Geometry check sheet. Reference: the model listing, model coordinates, mm. A direction names the side the tool comes from. Round coordinates to 2 decimals unless told otherwise and drop trailing zeros. Loops run counter-clockwise (first coordinate to the right, second up) from the corner with the lowest first, then second, coordinate; pieces in that order, holes last. Notation, with made-up numbers: (12.5, 49) - (27.5, 49) arc R21 ccw to (27.5, 79) - close; hole circle Ø9 at (76, -33.75). An arc over 180 degrees is marked (long way). Answer as CSV lines item,"result". Start each with the question number.
1) Cross-section at C-C on z = -7.1. Record the boundary of the cut face in (x, y) (3 decimals).
2) Cross-section at D-D on y = 5.5. Record the boundary of the cut face in (x, z), and give its area (3 significant figures).
3) Depth check by flat-ended pin: P1, Ø8, axis at y = 11.5, z = -7, coming from the -X side; P2, Ø3, axis at x = -1.5, z = 10.5, coming from the +Y side; P3, Ø1, axis at y = 3, z = -3.5, coming from the +X side; P4, Ø0.6, axis at x = -2, y = 3, coming from the -Z side. Enter the tip coordinate at first touch or a pass-through.
4) Draft check along Z on faces 4 (the cylindrical face through (-14.63, 1.01, 3.44)), 5 (the cylindrical face through (-13.887, 0.986, 10.648)), 6 (the flat face through (-4, 4, -4)). Enter one of: released by +Z, released by -Z, zero draft, split by the parting line, or undercut.
5) Cross-section at A-A on y = 3. Record the boundary of the cut face in (x, z), and give its area (3 significant figures).
6) Thickness scan on line 1 along Z through (x, y) = (-2, 2.1); line 2 along Z through (x, y) = (-13.5, 1.25); line 3 along X through (y, z) = (1.35, -4.1). Record the ranges inside material, lowest first.
7) Cross-section at B-B on y = 9. Record the boundary of the cut face in (x, z).
8) Access from +Z, -Z, +X, -X, +Y, -Y to the whole of each face (thin tool, end or side, straight path). Record for faces 1 (the cylindrical face through (-1, 3, -0.7)), 2 (the cylindrical face through (4.5, 9, 1.1)), 3 (the cylindrical face through (14.049, 1.014, 8.166)).
from build123d import *

# Parameters (mm, degrees)
SKETCH1_R                                       = 17.5
BOSS_EXTRUDE1_DEPTH                             = 2
CUT_EXTRUDE1_DEPTH                              = 3
CIRPATTERN1_COUNT                               = 6
SKETCH3_W                                       = 13.5
SKETCH3_H                                       = 16.4
BOSS_EXTRUDE2_DEPTH                             = 17.5
SKETCH4_W                                       = 13.5
SKETCH4_H                                       = 8.2
CUT_EXTRUDE2_DEPTH                              = 11.5
CUT_EXTRUDE3_DEPTH                              = 26.7
CUT_EXTRUDE4_DEPTH                              = 8.2
F_1_5MM_DOWEL_HOLE1_D                           = 1.5
F_1_5MM_DOWEL_HOLE1_DEPTH                       = 5
F_1_5MM_DOWEL_HOLE1_TIP                         = 0.450645464
F_1_5MM_DOWEL_HOLE2_D                           = 1.5
F_1_5MM_DOWEL_HOLE2_DEPTH                       = 3
F_1_5MM_DOWEL_HOLE2_TIP                         = 0.450645464
F_1_5MM_DOWEL_HOLE4_D                           = 1.5
F_1_5MM_DOWEL_HOLE4_DEPTH                       = 5
F_1_5MM_DOWEL_HOLE4_TIP                         = 0.450645464
F_1_5MM_DOWEL_HOLE3_D                           = 1.5
F_1_5MM_DOWEL_HOLE3_DEPTH                       = 5
F_1_5MM_DOWEL_HOLE3_TIP                         = 0.450645464
SKETCH16_R                                      = 1
CUT_EXTRUDE7_DEPTH                              = 14.5
CSK_FOR_M2_FLAT_HEAD_MACHINE_SCREW2_D           = 2.4
CSK_FOR_M2_FLAT_HEAD_MACHINE_SCREW2_CSINK_D     = 4.4
CSK_FOR_M2_FLAT_HEAD_MACHINE_SCREW2_CSINK_ANGLE = 90
CUT_EXTRUDE6_DEPTH                              = 11.5


with BuildPart() as part:
    # Sketch1 → Boss-Extrude1 (new body)
    with BuildSketch(Plane(origin=(0, 0, 0), x_dir=(1, 0, 0), z_dir=(0, 1, 0))):
        Circle(SKETCH1_R)
    extrude(amount=BOSS_EXTRUDE1_DEPTH)

    # Sketch2 → Cut-Extrude1 (cut, through all)
    with BuildSketch(Plane(origin=(0, 2, 0), x_dir=(1, 0, 0), z_dir=(0, 1, 0))):
        with BuildLine():
            ThreePointArc((3.378564976, 15.894898512), (0, 16.25), (-3.378564976, 15.894898512))
            ThreePointArc((-3.378564976, 15.894898512), (-4.341359863, 14.412324397), (-2.858785749, 13.44952951))
            ThreePointArc((-2.858785749, 13.44952951), (0, 13.75), (2.858785749, 13.44952951))
            ThreePointArc((2.858785749, 13.44952951), (4.341359863, 14.412324397), (3.378564976, 15.894898512))
        make_face()
    cut_extrude1 = extrude(amount=-CUT_EXTRUDE1_DEPTH, mode=Mode.SUBTRACT)

    # CirPattern1: Cut-Extrude1 ×6 about axis
    cirpattern1_axis = Axis((0, 0, 0), (0, 1, 0))
    for i in range(1, CIRPATTERN1_COUNT):
        add(cut_extrude1.rotate(cirpattern1_axis, i * 360 / CIRPATTERN1_COUNT), mode=Mode.SUBTRACT)

    # Sketch3 → Boss-Extrude2 (add)
    with BuildSketch(Plane(origin=(0, 2, 0), x_dir=(1, 0, 0), z_dir=(0, 1, 0))):
        Rectangle(SKETCH3_W, SKETCH3_H)
    extrude(amount=BOSS_EXTRUDE2_DEPTH)

    # Sketch4 → Cut-Extrude2 (cut)
    with BuildSketch(Plane(origin=(0, 19.5, 0), x_dir=(1, 0, 0), z_dir=(0, 1, 0))):
        with Locations((0, 4.1)):
            Rectangle(SKETCH4_W, SKETCH4_H)
    extrude(amount=-CUT_EXTRUDE2_DEPTH, mode=Mode.SUBTRACT)

    # Sketch5 → Cut-Extrude3 (cut, through all)
    with BuildSketch(Plane.XY.offset(8.2)):
        Polygon((-6.75, 19.5), (-6.75, 13.5), (0, 13.5), (0, 10.5), (6.75, 10.5), (6.75, 19.5), align=None)
    extrude(amount=-CUT_EXTRUDE3_DEPTH, mode=Mode.SUBTRACT)

    # Sketch6 → Cut-Extrude4 (cut)
    with BuildSketch(Plane(origin=(0, 0, -8.2), x_dir=(-1, 0, 0), z_dir=(0, 0, -1))):
        Polygon((6.75, 8), (6.75, 4), (0, 4), (0, 2), (-6.75, 2), (-6.75, 8), align=None)
    extrude(amount=-CUT_EXTRUDE4_DEPTH, mode=Mode.SUBTRACT)

    # Ø1.5mm Dowel Hole1
    with Locations(Plane(origin=(0, 13.5, 0), x_dir=(1, 0, 0), z_dir=(0, 1, 0))):
        with Locations((-2, -1.1), (-2, -7.1)):
            Hole(F_1_5MM_DOWEL_HOLE1_D / 2, depth=F_1_5MM_DOWEL_HOLE1_DEPTH)
            with Locations((0, 0, -(F_1_5MM_DOWEL_HOLE1_DEPTH + F_1_5MM_DOWEL_HOLE1_TIP / 2))):  # 118° drill point
                Cone(0, F_1_5MM_DOWEL_HOLE1_D / 2, F_1_5MM_DOWEL_HOLE1_TIP, mode=Mode.SUBTRACT)

    # Ø1.5mm Dowel Hole2
    with Locations(Plane(origin=(0, 10.5, 0), x_dir=(1, 0, 0), z_dir=(0, 1, 0))):
        with Locations((3.75, -1.1), (3.75, -7.1)):
            Hole(F_1_5MM_DOWEL_HOLE2_D / 2, depth=F_1_5MM_DOWEL_HOLE2_DEPTH)
            with Locations((0, 0, -(F_1_5MM_DOWEL_HOLE2_DEPTH + F_1_5MM_DOWEL_HOLE2_TIP / 2))):  # 118° drill point
                Cone(0, F_1_5MM_DOWEL_HOLE2_D / 2, F_1_5MM_DOWEL_HOLE2_TIP, mode=Mode.SUBTRACT)

    # Ø1.5mm Dowel Hole4
    with Locations(Plane(origin=(0, 4, 0), x_dir=(1, 0, 0), z_dir=(0, 1, 0))):
        with Locations((-2, 7.1), (-2, 1.1)):
            Hole(F_1_5MM_DOWEL_HOLE4_D / 2, depth=F_1_5MM_DOWEL_HOLE4_DEPTH)
            with Locations((0, 0, -(F_1_5MM_DOWEL_HOLE4_DEPTH + F_1_5MM_DOWEL_HOLE4_TIP / 2))):  # 118° drill point
                Cone(0, F_1_5MM_DOWEL_HOLE4_D / 2, F_1_5MM_DOWEL_HOLE4_TIP, mode=Mode.SUBTRACT)

    # Ø1.5mm Dowel Hole3
    with Locations(Plane(origin=(0, 2, 0), x_dir=(1, 0, 0), z_dir=(0, 1, 0))):
        with Locations((3.75, 7.1), (3.75, 1.1)):
            Hole(F_1_5MM_DOWEL_HOLE3_D / 2, depth=F_1_5MM_DOWEL_HOLE3_DEPTH)
            with Locations((0, 0, -(F_1_5MM_DOWEL_HOLE3_DEPTH + F_1_5MM_DOWEL_HOLE3_TIP / 2))):  # 118° drill point
                Cone(0, F_1_5MM_DOWEL_HOLE3_D / 2, F_1_5MM_DOWEL_HOLE3_TIP, mode=Mode.SUBTRACT)

    # Sketch16 → Cut-Extrude7 (cut, through all)
    with BuildSketch(Plane(origin=(0, 13.5, 0), x_dir=(1, 0, 0), z_dir=(0, 1, 0))):
        with Locations((-2, -4.1)):
            Circle(SKETCH16_R)
        with Locations((3.75, -4.1)):
            Circle(SKETCH16_R)
        with Locations((3.75, 4.1)):
            Circle(SKETCH16_R)
        with Locations((-2, 4.1)):
            Circle(SKETCH16_R)
    extrude(amount=-CUT_EXTRUDE7_DEPTH, mode=Mode.SUBTRACT)

    # CSK for M2 Flat Head Machine Screw2 (through all)
    with Locations(Plane(origin=(0, 0, 0), x_dir=(-1, 0, 0), z_dir=(0, -1, 0))):
        with Locations((-3.75, 4.1), (2, 4.1), (2, -4.1), (-3.75, -4.1)):
            CounterSinkHole(CSK_FOR_M2_FLAT_HEAD_MACHINE_SCREW2_D / 2, CSK_FOR_M2_FLAT_HEAD_MACHINE_SCREW2_CSINK_D / 2, counter_sink_angle=CSK_FOR_M2_FLAT_HEAD_MACHINE_SCREW2_CSINK_ANGLE)

    # Sketch19 → Cut-Extrude6 (cut)
    with BuildSketch(Plane(origin=(0, 2, 0), x_dir=(1, 0, 0), z_dir=(0, 1, 0))):
        with BuildLine():
            Line((-0.25, 1.5), (1.22977385, 1.5))
            ThreePointArc((1.22977385, 1.5), (1.97977385, 0.75), (1.22977385, 0))
            Line((1.22977385, 0), (-0.25, 0))
            ThreePointArc((-0.25, 0), (-1, 0.75), (-0.25, 1.5))
        make_face()
    extrude(amount=CUT_EXTRUDE6_DEPTH, mode=Mode.SUBTRACT)


solid = part.part
Answer block:
1,outline,"(-15.995, 0) - (-14.617, 0) - (-14.617, 2) - (-15.995, 2) - close; (-11.775, 0) - (-2.75, 0) - (-2.75, 4) - (-6.75, 4) - (-6.75, 2) - (-11.775, 2) - close; (-1.25, 0) - (3, 0) - (3, 2) - (0, 2) - (0, 4) - (-1.25, 4) - close; (4.5, 0) - (11.775, 0) - (11.775, 2) - (4.5, 2) - close; (14.617, 0) - (15.995, 0) - (15.995, 2) - (14.617, 2) - close"
2,outline,"(-6.75, 0) - (6.75, 0) - (6.75, 8.2) - (-6.75, 8.2) - close; hole circle Ø2.4 at (-2, 4.1); hole circle Ø2.4 at (3.75, 4.1)"
2,area,"102 mm^2"
3,P1,"passes through"
3,P2,"stops at y = 2"
3,P3,"stops at x = 0"
3,P4,"stops at z = -8.2"
4,face 4,"undercut"
4,face 5,"split by the parting line"
4,face 6,"zero draft"
5,outline,"(-6.75, -8.2) - (0, -8.2) - (0, -1.5) - (-0.25, -1.5) arc R0.75 cw to (-0.25, 0) - (6.75, 0) - (6.75, 8.2) - (-6.75, 8.2) - close; hole circle Ø2.4 at (-2, -4.1); hole circle Ø2.4 at (-2, 4.1); hole circle Ø1.5 at (-2, -7.1); hole circle Ø1.5 at (-2, -1.1); hole circle Ø2.4 at (3.75, 4.1)"
5,area,"148 mm^2"
6,line 1,"z = -8.2 to -7.85, -6.35 to -5.3, -2.9 to -1.85, -0.35 to 2.9, 5.3 to 8.2"
6,line 2,"z = -11.14 to -9.05, -3.65 to 3.65, 9.05 to 11.14"
6,line 3,"x = -17.01 to -15.4, -13.14 to -3.2, -0.8 to 2.55, 4.95 to 13.14, 15.4 to 17.01"
7,outline,"(-6.75, 0) - (6.75, 0) - (6.75, 8.2) - (-6.75, 8.2) - close; hole circle Ø2.4 at (-2, 4.1); hole circle Ø1.5 at (-2, 1.1); hole circle Ø1.5 at (-2, 7.1); hole circle Ø2.4 at (3.75, 4.1); hole circle Ø1.5 at (3.75, 1.1); hole circle Ø1.5 at (3.75, 7.1)"
8,face 1,"+X, +Y"
8,face 2,"+Y"
8,face 3,"+Y, -Y"
